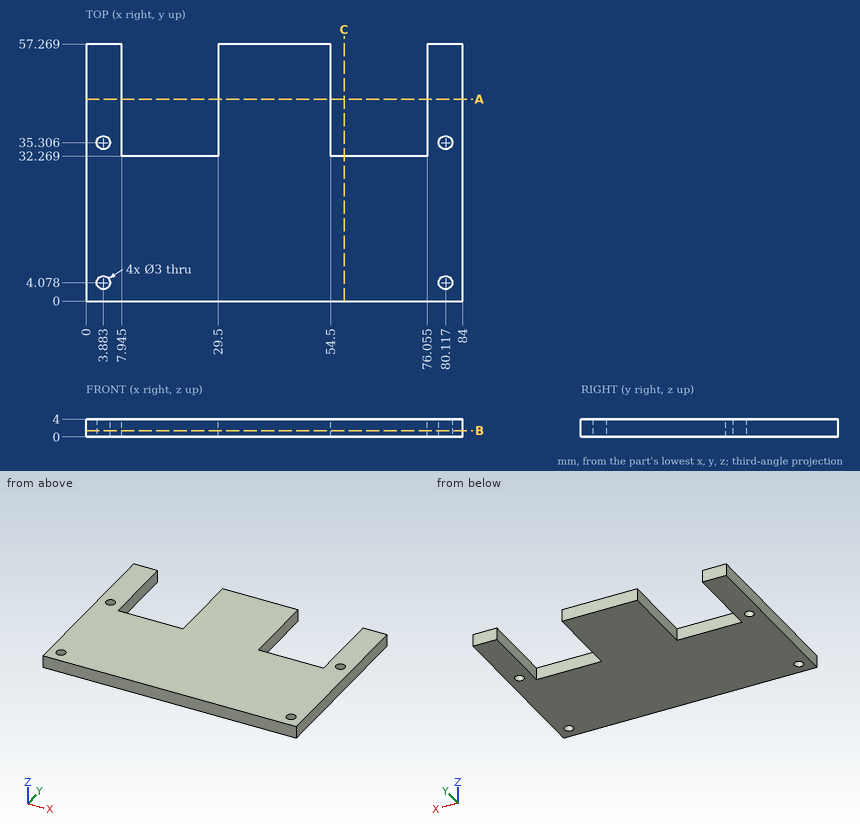
Study the drawing (mm; zero at the part's minimum x, y, z) and answer. Coordinates: 2 decimals unless noted, no trailing zeros. Write each loop counter-clockwise with the first axis right and the second up, starting at its lowest first coordinate (ties: lowest second). Pieces come first, ordered by that corner, then holes. Notation, with made-up numbers: (51.25, -15.75) - (62.25, -15.75) arc R32 cw to (62.25, 19.25) - close; hole circle Ø2 at (2.25, 42). An arc over 180 degrees is marked (long way). Answer as a JSON object with one key per item and string values. Group by question number.
1. A cutting plane is placed at B-B (z = 1.4). Determine the outline of the cut face in (x, y) (1 decimal).
2. This flat-tipped pin is pushed along its axis until it touches: P1, Ø1.5, axis at x = 59.5, z = 3, coming from the +Y side. Where does it stop, or does it pass through?
3. A cutting plane is placed at C-C (x = 57.5). Determine the outline of the cut face in (y, z), plus the area to 3 significant figures.
4. A cutting plane is placed at A-A (y = 45). Determine the outline of the cut face in (x, z) (1 decimal).
5. Consider L1, parallel to X at y = 53, z = 2.95 (1 decimal); L2, parallel to X at y = 4, z = 3.45 (1 decimal); L3, parallel to X at y = 35.5, z = 2.8 (1 decimal). Determine where each line is inside the solid, lowest interval first. Write a range as [from, to].
Worked out:
{
 "1": {"outline": "(0, 0) - (84, 0) - (84, 57.3) - (76.1, 57.3) - (76.1, 32.3) - (54.5, 32.3) - (54.5, 57.3) - (29.5, 57.3) - (29.5, 32.3) - (7.9, 32.3) - (7.9, 57.3) - (0, 57.3) - close; hole circle Ø3 at (3.9, 4.1); hole circle Ø3 at (3.9, 35.3); hole circle Ø3 at (80.1, 4.1); hole circle Ø3 at (80.1, 35.3)"},
 "2": {"P1": "stops at y = 32.27"},
 "3": {"outline": "(0, 0) - (32.27, 0) - (32.27, 4) - (0, 4) - close", "area": "129 mm²"},
 "4": {"outline": "(0, 0) - (7.9, 0) - (7.9, 4) - (0, 4) - close; (29.5, 0) - (54.5, 0) - (54.5, 4) - (29.5, 4) - close; (76.1, 0) - (84, 0) - (84, 4) - (76.1, 4) - close"},
 "5": {"L1": "x = [0, 7.9], [29.5, 54.5], [76.1, 84]", "L2": "x = [0, 2.4], [5.4, 78.6], [81.6, 84]", "L3": "x = [0, 2.4], [5.4, 7.9], [29.5, 54.5], [76.1, 78.6], [81.6, 84]"}
}
